Verification items for the finished model (mm, model axes). Give positions to 0.01 mm unless a question says otherwise; leave off trailing zeros. Loops run counter-clockwise (first coordinate to the right, second up) from the corner with the lowest first, then second, coordinate; pieces in that order, holes last. Notation, with made-up numbers: M -6,47 L 33,47 A28 ccw 33,83 Z; hole C 12.5,56.5 d6. An arc over 180 degrees is marked long. Use CSV: the item, a comma, the result in double quotes.
Autodesk Inventor part; units mm, degrees
ref_plane "YZ Plane" through (0, 0, 0) normal (1, 0, 0) x (0, 1, 0)
ref_plane "XZ Plane" through (0, 0, 0) normal (0, 1, 0) x (-1, 0, 0)
ref_plane "XY Plane" through (0, 0, 0) normal (0, 0, 1) x (1, 0, 0)
sketch "Szkic1" plane through (0, 0, 0) normal (0, 0, 1) x (1, 0, 0)
  line L0 (144, 100) -> (-144, 100)
  line L1 (-144, 100) -> (-144, -100)
  line L2 (-144, -100) -> (144, -100)
  line L3 (144, -100) -> (144, 100)
  line L4 (144, 100) -> (-144, -100) construction
  line L5 (-144, 100) -> (144, -100) construction
  point P0 (0, 0)
  dimension "d0" = 288
  dimension "d1" = 200
extrude "Wyciągnięcie proste1" add sketch "Szkic1" along normal mid plane 6
sketch "Szkic2" plane through (0, 0, -3) normal (0, 0, -1) x (-1, 0, 0)
  line L0 (11, 51) -> (-11, 51)
  line L1 (-11, 51) -> (-11, 85)
  line L2 (-11, 85) -> (11, 85)
  line L3 (11, 85) -> (11, 51)
  line L4 (11, 51) -> (-11, 85) construction
  line L5 (-11, 51) -> (11, 85) construction
  line L6 (144, 100) -> (-144, 100)
  line L7 (-144, 100) -> (-144, -100)
  circle A0 centre (0, 73) radius 10.5
  line L8 (-144, -100) -> (144, -100)
  line L9 (144, -100) -> (144, 100)
  line L10 (-5, 51) -> (-5, -100)
  line L11 (5, 51) -> (5, -100)
  point P0 (0, 0)
  point P1 (0, 68)
  dimension "d4" = 34
  dimension "d5" = 22
  dimension "d6" = 15
  dimension "d8" = 21
  dimension "d9" = 12
  dimension "d10" = 11
  dimension "d15" = 10
  dimension "d16" = 139
  dimension "d19" = 144
extrude "Wyciągnięcie proste2" cut sketch "Szkic2" against normal through all contours A0
extrude "Wyciągnięcie proste3" cut sketch "Szkic2" against normal blind 3 contours L0 L1 L2 L3
extrude "Wyciągnięcie proste5" cut sketch "Szkic2" against normal blind 3 contours L11 L8 L10 L0
properties part number "RightWall"
(1) Section check A-A on y = 73. Record the cut outline in (x, z), plus the area to 3 significant figures.
Calculated:
outline,"M -144,-3 L -11,-3 L -11,0 L -10.5,0 L -10.5,3 L -144,3 Z; M 10.5,0 L 11,0 L 11,-3 L 144,-3 L 144,3 L 10.5,3 Z"
area,"1,600 mm²"
(2) Depth check by flat-ended pin: pin 1 Ø2.5 at (x, z) = (-4.5, -1) entering from -Y; pin 2 Ø6.5 at (x, y) = (1, 19.5) entering from -Z. Enter the tip coordinate at first touch or a pass-through.
Calculated:
pin 1,"stops at y = -100"
pin 2,"stops at z = 0"
(3) Scan lines: L1, parallel to X at y = 5.5, z = -1.75; L2, parallel to Y at x = 0, z = 1.6; L3, parallel to Z at x = 10.5, y = 74. Record each from-to range of solid material in increasing order. Write a range as from..to.
Calculated:
L1,"x = -144..-5, 5..144"
L2,"y = -100..62.5, 83.5..100"
L3,"z = 0..3"
(4) Section check B-B on x = 0. Record the cut outline in (y, z).
Calculated:
outline,"M -100,0 L 62.5,0 L 62.5,3 L -100,3 Z; M 83.5,0 L 85,0 L 85,-3 L 100,-3 L 100,3 L 83.5,3 Z"
(5) Section check D-D on y = 29. Record the cut outline in (x, z).
Calculated:
outline,"M -144,-3 L -5,-3 L -5,0 L 5,0 L 5,-3 L 144,-3 L 144,3 L -144,3 Z"
(6) Mould release check, pull along Y, two halves, no side actions. Record for faces 1 (the cylindrical face through (1.37, 83.41, 1.48)), 2 (the flat face through (-144, 1, 0)), 3 (the flat face through (2, 100, 0)): released by +Y, released by -Y, zero draft, split by the parting line, or undercut.
Calculated:
face 1,"undercut"
face 2,"zero draft"
face 3,"released by +Y"
(7) Section check C-C on z = -1.45. Record the cut outline in (x, y), plus the area to 3 significant figures.
Calculated:
outline,"M -144,-100 L -5,-100 L -5,51 L -11,51 L -11,85 L 11,85 L 11,51 L 5,51 L 5,-100 L 144,-100 L 144,100 L -144,100 Z"
area,"55,300 mm²"
